Here's the drawing with two shaded views (mm, measured from the low corner). I have some questions. A direction names the side the tool comes from. Round coordinates to 2 decimals unless told otherwise and drop trailing zeros. Loops run counter-clockwise (first coordinate to the right, second up) from the corner with the lowest first, then second, coordinate; pieces in that order, holes last. Notation, with made-up numbers: (48.5, -25) -> (72.5, -25) arc R9 cw to (72.5, -20) -> close; hole circle Ø3 at (-17, 54). An arc over 180 degrees is marked (long way). Write each question's results on one line, items separated by ' | '.
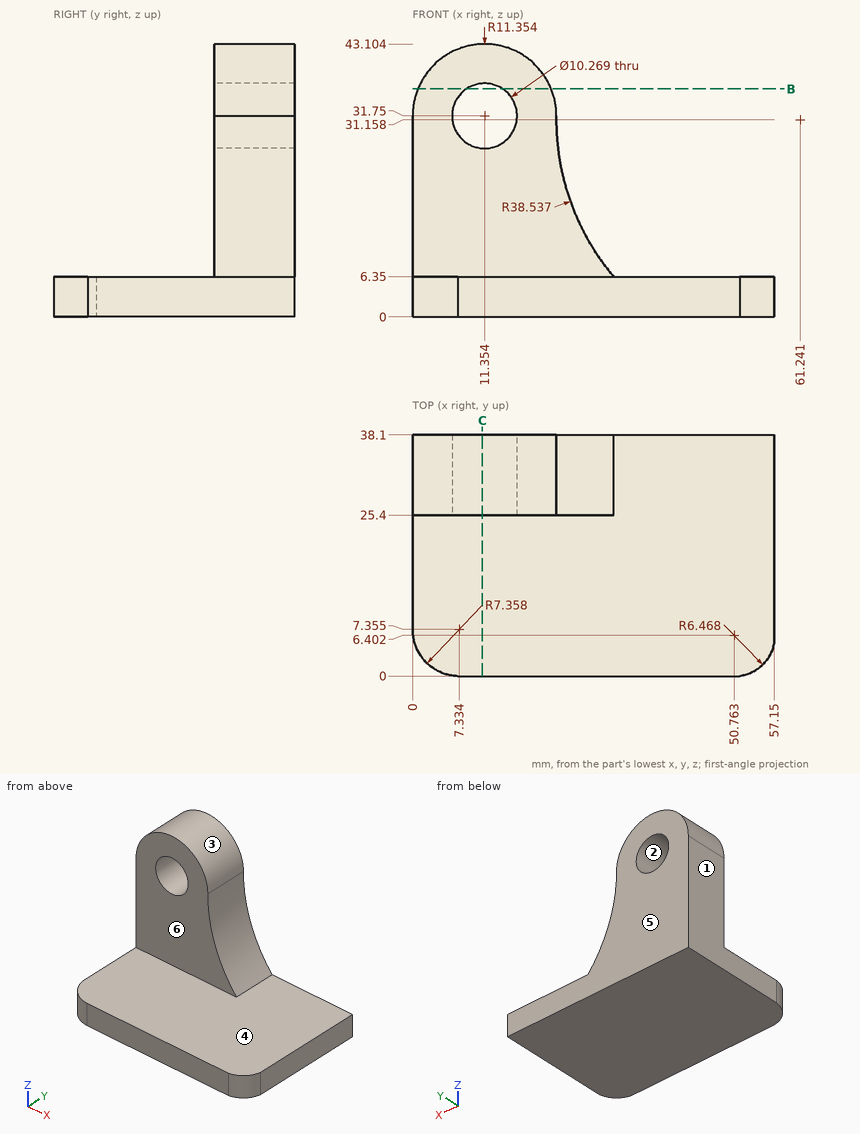
1. Will these pins go through, and if not, where does the flat tip stop? pin 1 (12 mm diameter, centred on x = 38, y = 24.5, fed in from +Z); pin 2 (13.5 mm diameter, centred on x = 11.35, z = 31.75, fed in from -Y).
Final values:
pin 1: z = 6.35 | pin 2: y = 25.4
2. Please list where these lines run through material, in increasing order: line 1 (Y direction, x = 22, z = 15); line 2 (Z direction, x = 14.5, y = 12.5); line 3 (X direction, y = 29, z = 31) (1 decimal). Write a range as from..to.
Final values:
line 1: 25.4..38.1 | line 2: 0..6.35 | line 3: 0..6.3, 16.4..22.7
3. If we section it at B-B (z = 36): List the corners of the cut face in (x, y) for me (1 decimal).
Final values:
outline: (0.8, 25.4) -> (8.5, 25.4) -> (8.5, 38.1) -> (0.8, 38.1) -> close; (14.2, 25.4) -> (21.9, 25.4) -> (21.9, 38.1) -> (14.2, 38.1) -> close
4. On a 3-axis mill with a long thin cutter (end or side, diameter ignored), from which of +Z, -Z, +X, -X, +Y, -Y can I reach the whole of each face in a straight line? I mean the marked faces 4, 5 and 6. Say none if no direction works.
Final values:
face 4: +Z, +X, -Y | face 5: +Z, -Z, +X, -X, +Y | face 6: +Z, +X, -X, -Y
5. If we section it at C-C (x = 11): List the corners of the cut face in (y, z) for me.
Final values:
outline: (0, 0) -> (38.1, 0) -> (38.1, 26.63) -> (25.4, 26.63) -> (25.4, 6.35) -> (0, 6.35) -> close; (25.4, 36.87) -> (38.1, 36.87) -> (38.1, 43.1) -> (25.4, 43.1) -> close
6. We'd pull the mould along Z, two halves only. Please class the marked faces 1, 2 and 3: pulls with the +Z half, pulls with the -Z half, needs draft (parallel to the pull), parting line crosses it, or undercut.
Final values:
face 1: needs draft | face 2: undercut | face 3: pulls with the +Z half
